Design review of the part built by this model. Coordinates are the model's own, in mm. A direction names the side the tool comes from. Coordinates: 2 decimals unless noted, no trailing zeros. Loops run counter-clockwise (first coordinate to the right, second up) from the corner with the lowest first, then second, coordinate; pieces in that order, holes last. Notation, with made-up numbers: (-27.75, 36) - (-22.75, 36) arc R17 cw to (-22.75, 62) - close; hole circle Ø3 at (71, 67.5). An arc over 180 degrees is marked (long way). Answer in a Markdown table with one row per item. Add a question column.
(1) We need section C-C, the plane y = -5.5. Write out the cut boundary in (x, z), plus the area to 4 significant figures.
(2) The part is to be moulded in two halves that separate along Y. For faces 1 (the face through (32.6, -13, 2)), 2 (the face through (23, 22.5, 2)), 3 (the face through (1.5, -10, 2)), say which applies: released by +Y, released by -Y, zero draft, split by the parting line, or undercut.
(3) We need section D-D, the plane y = -10. Write out the cut boundary in (x, z).
(4) We need section A-A, the plane y = 13. Write out the cut boundary in (x, z).
(5) For faces 4 (the face through (2.6, 13, 2)), 5 (the face through (35, 20, 2)), 6 (the face through (28.5, -10, 2)), list the 3-axis set-ups (+Z, -Z, +X, -X, +Y, -Y) from which the entire face can be reached by the end or side of a thin tool; tool diameter is ignored.
(6) To check wall thickness, follow L1, parallel to X at y = 10, z = 3.6; L2, parallel to X at y = 20.5, z = 3.45; L3, parallel to Y at x = 15, z = 3.3. State the ranges of each line that lie inside material, in increasing order. Write a range as [from, to].
(7) We need section B-B, the plane x = 15. Write out the cut boundary in (y, z), plus the area to 4 significant figures.
(8) Clearance check with flat-ended pins moving along their axes: pin 1 (1.2 mm diameter, centred on x = 28, z = 1.5, fed in from +Y); pin 2 (0.6 mm diameter, centred on x = 2, z = 1.5, fed in from -Y). State where each tip first meets the part, or that it passes through.
from build123d import *

# Parameters (mm, degrees)
ESQUISSE1_R        = 4.25
BOSS_EXTRU_1_DEPTH = 5


with BuildPart() as part:
    # Esquisse1 → Boss.-Extru.1 (new body)
    # profile 1 of 2: a face of its own
    with BuildSketch(Plane.XY):
        Polygon((-10, 22.5), (-10, 17.5), (-10, -17.5), (-10, -22.5), (-5, -22.5), (-5, -17.5), (-1.5, -17.5), (-1.5, -14.5), (-2.6, -14.5), (-2.6, -12.2), (-1.5, -12.2), (-1.5, -7.5), (1.5, -7.5), (1.5, -12.2), (2.6, -12.2), (2.6, -14.5), (1.5, -14.5), (1.5, -17.5), (5, -17.5), (5, -22.5), (10, -22.5), (10, -17.5), (10, 17.5), (10, 22.5), (5, 22.5), (5, 17.5), (1.5, 17.5), (1.5, 14.5), (2.6, 14.5), (2.6, 12.2), (1.5, 12.2), (1.5, 7.5), (-1.5, 7.5), (-1.5, 12.2), (-2.6, 12.2), (-2.6, 14.5), (-1.5, 14.5), (-1.5, 17.5), (-5, 17.5), (-5, 22.5), align=None)
    # profile 2 of 2: a face of its own
    with BuildSketch(Plane.XY):
        Polygon((20, 17.5), (10, 17.5), (10, -17.5), (20, -17.5), (20, -22.5), (25, -22.5), (25, -17.5), (28.5, -17.5), (28.5, -14.5), (27.4, -14.5), (27.4, -12.2), (28.5, -12.2), (28.5, -7.5), (31.5, -7.5), (31.5, -12.2), (32.6, -12.2), (32.6, -14.5), (31.5, -14.5), (31.5, -17.5), (35, -17.5), (35, -22.5), (40, -22.5), (40, -17.5), (40, 17.5), (40, 22.5), (35, 22.5), (35, 17.5), (31.5, 17.5), (31.5, 14.5), (32.6, 14.5), (32.6, 12.2), (31.5, 12.2), (31.5, 7.5), (28.5, 7.5), (28.5, 12.2), (27.4, 12.2), (27.4, 14.5), (28.5, 14.5), (28.5, 17.5), (25, 17.5), (25, 22.5), (20, 22.5), align=None)
        with Locations((15, -7.5)):
            Circle(ESQUISSE1_R, mode=Mode.SUBTRACT)
    extrude(amount=BOSS_EXTRU_1_DEPTH)


solid = part.part
Responses:
| question | item | result |
|---|---|---|
| 1 | outline | (-10, 0) - (11.25, 0) - (11.25, 5) - (-10, 5) - close; (18.75, 0) - (40, 0) - (40, 5) - (18.75, 5) - close |
| 1 | area | 212.5 mm2 |
| 2 | face 1 | undercut |
| 2 | face 2 | released by +Y |
| 2 | face 3 | zero draft |
| 3 | outline | (-10, 0) - (-1.5, 0) - (-1.5, 5) - (-10, 5) - close; (1.5, 0) - (11.56, 0) - (11.56, 5) - (1.5, 5) - close; (18.44, 0) - (28.5, 0) - (28.5, 5) - (18.44, 5) - close; (31.5, 0) - (40, 0) - (40, 5) - (31.5, 5) - close |
| 4 | outline | (-10, 0) - (-2.6, 0) - (-2.6, 5) - (-10, 5) - close; (2.6, 0) - (27.4, 0) - (27.4, 5) - (2.6, 5) - close; (32.6, 0) - (40, 0) - (40, 5) - (32.6, 5) - close |
| 5 | face 4 | +Z, -Z |
| 5 | face 5 | +Z, -Z, +Y |
| 5 | face 6 | +Z, -Z, -Y |
| 6 | L1 | x = [-10, -1.5], [1.5, 28.5], [31.5, 40] |
| 6 | L2 | x = [-10, -5], [5, 10], [20, 25], [35, 40] |
| 6 | L3 | y = [-17.5, -11.75], [-3.25, 17.5] |
| 7 | outline | (-17.5, 0) - (-11.75, 0) - (-11.75, 5) - (-17.5, 5) - close; (-3.25, 0) - (17.5, 0) - (17.5, 5) - (-3.25, 5) - close |
| 7 | area | 132.5 mm2 |
| 8 | pin 1 | stops at y = 17.5 |
| 8 | pin 2 | stops at y = -17.5 |
